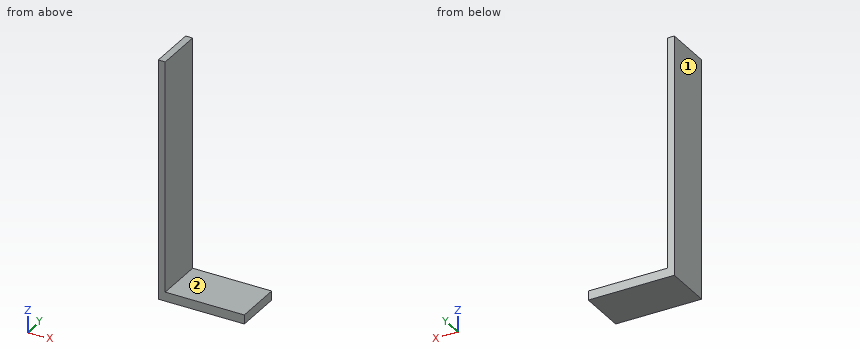
from build123d import *

# Parameters (mm, degrees)
F3_DEPTH = 12.7


# Not quite as in the source:
# - the program builds the solid bodies; features that only make, move or delete a surface that nothing else refers to are left out


with BuildPart() as f3:
    # F2 (on Front) → F3 (new body, symmetric)
    with BuildSketch(Plane.XZ):
        Polygon((59.2198967934, 63.1065145135), (55.5164813995, 63.1065145135), (55.5164813995, -59.8734021187), (55.5164813995, -64.7067055106), (101.3612598181, -64.7067055106), (101.3612598181, -59.8734021187), (59.2198967934, -59.8734021187), align=None)
    extrude(amount=F3_DEPTH, both=True)


solid = f3.part
Input: part model. Units: mm. Frame: model coordinates. Face numbers are marked on the shaded views. A direction names the side the tool comes from. Give positions to 0.01 mm unless a question says otherwise; leave off trailing zeros. Order: outer loops, then holes, each group sorted by start corner. A loop starts at its lowest first (then second) coordinate and runs counter-clockwise, first axis right, second up. Notation, with made-up numbers: M 56,41.5 L 98,41.5 A19 ccw 98,61.5 Z; hole C 17.25,37 d9. An arc over 180 degrees is marked long. Answer as a JSON object with one key per item and string values.
1. First-contact query: P1, Ø7.5, axis at y = 0.5, z = 18, coming from the +X side; P2, Ø4, axis at x = 80, y = 9.5, coming from the +Z side. Flat tips, straight axial feed; report the tip coordinate or a pass-through.
Result sheet:
{"P1": "x = 59.22", "P2": "z = -59.87"}
2. Ray query, line 1 (X direction, y = -4.5, z = -41.5); line 2 (Z direction, x = 62.5, y = 6.75). Return the intervals inside material, ascending. Write a range as [from, to].
Result sheet:
{"line 1": "[55.52, 59.22]", "line 2": "[-64.71, -59.87]"}
3. Cut plane C-C, the plane x = 72. Output: boundary loops of the cut face in (y, z).
Result sheet:
{"outline": "M -12.7,-64.71 L 12.7,-64.71 L 12.7,-59.87 L -12.7,-59.87 Z"}
4. Cut plane B-B, the plane z = -49.5. Output: boundary loops of the cut face in (x, y).
Result sheet:
{"outline": "M 55.52,-12.7 L 59.22,-12.7 L 59.22,12.7 L 55.52,12.7 Z"}
5. Cut plane A-A, the plane y = -5. Output: boundary loops of the cut face in (x, z).
Result sheet:
{"outline": "M 55.52,-64.71 L 101.36,-64.71 L 101.36,-59.87 L 59.22,-59.87 L 59.22,63.11 L 55.52,63.11 Z"}
6. Reachability of the marked faces 1 and 2 from +Z, -Z, +X, -X, +Y, -Y: full face, straight path, thin tool, end or side. Return the list, or none.
Result sheet:
{"face 1": "+Z, -Z, -X, +Y, -Y", "face 2": "+Z, +X, +Y, -Y"}
